Verification items for the finished model (mm, model axes). Face numbers are marked on the shaded views. A direction names the side the tool comes from. Give positions to 0.01 mm unless a question says otherwise; leave off trailing zeros. Write each loop counter-clockwise with the first axis right and the second up, starting at its lowest first coordinate (ties: lowest second). Pieces come first, ordered by that corner, then holes. Notation, with made-up numbers: M 4.5,-17.5 L 31.5,-17.5 A20 ccw 31.5,-11.5 Z; hole C 61,39.5 d3. An arc over 180 degrees is marked long. Write item = value, one per line.
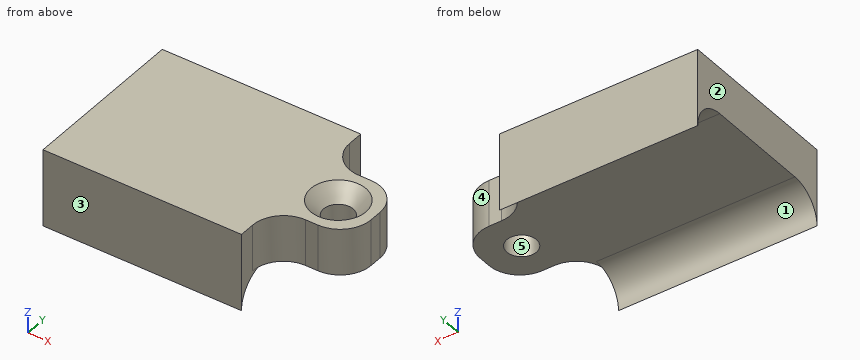
from build123d import *

# Parameters (mm, degrees)
SKETCH1_W                       = 12.8
SKETCH1_H                       = 10.8
SKETCH1_W_2                     = 4.8
SKETCH1_H_2                     = 4.8
BOSS_EXTRUDE1_DEPTH             = 1.5
F_2_CLEARANCE_HOLE1_D           = 1.905
F_2_CLEARANCE_HOLE1_CSINK_D     = 3.556
F_2_CLEARANCE_HOLE1_CSINK_ANGLE = 80
FILLET1_R                       = 2
BOSS_EXTRUDE2_REACH             = 14.524
BOSS_EXTRUDE2_DIRECTION_2_REACH = 14.524


with BuildPart() as part:
    # Sketch1 → Boss-Extrude1 (new, symmetric)
    with BuildSketch(Plane.XY):
        Rectangle(SKETCH1_W, SKETCH1_H)
        with Locations((8.8, 0)):
            Rectangle(SKETCH1_W_2, SKETCH1_H_2)
    extrude(amount=BOSS_EXTRUDE1_DEPTH, both=True)

    # #2 Clearance Hole1 (through all)
    with Locations(Plane.XY.offset(1.5)):
        with Locations((8.8, 0)):
            CounterSinkHole(F_2_CLEARANCE_HOLE1_D / 2, F_2_CLEARANCE_HOLE1_CSINK_D / 2, counter_sink_angle=F_2_CLEARANCE_HOLE1_CSINK_ANGLE)

    # Fillet1
    fillet1_edges = [part.edges().sort_by_distance(p)[0] for p in [
        (6.4, 2.4, 0),
        (11.2, 2.4, 0),
        (11.2, -2.4, 0),
        (6.4, -2.4, 0),
    ]]
    fillet(fillet1_edges, radius=FILLET1_R)

    # Boss-Extrude2: up to this face of the body (flat: up to its plane)
    boss_extrude2_end = Plane(part.part.faces().sort_by_distance((-6.4, 0, 0))[0])
    # Sketch4 → Boss-Extrude2 (add, up to the picked face)
    with BuildSketch(Plane(origin=(0, 0, 0), x_dir=(0, 0, -1), z_dir=(1, 0, 0)), mode=Mode.PRIVATE) as boss_extrude2_sk1:
        with BuildLine():
            Line((1.5, 5.4), (3.5, 5.4))
            ThreePointArc((3.5, 5.4), (2.085786438, 4.814213562), (1.5, 3.4))
            Line((1.5, 3.4), (1.5, 5.4))
        make_face()
    boss_extrude2_tool1 = split(extrude(boss_extrude2_sk1.sketch, amount=-BOSS_EXTRUDE2_REACH, mode=Mode.PRIVATE), bisect_by=boss_extrude2_end, keep=Keep.BOTH, mode=Mode.PRIVATE)
    # Sketch4 → Boss-Extrude2 (add, up to the picked face)
    with BuildSketch(Plane(origin=(0, 0, 0), x_dir=(0, 0, -1), z_dir=(1, 0, 0)), mode=Mode.PRIVATE) as boss_extrude2_sk2:
        with BuildLine():
            Line((1.5, -5.4), (1.5, -3.4))
            ThreePointArc((1.5, -3.4), (2.085786438, -4.814213562), (3.5, -5.4))
            Line((3.5, -5.4), (1.5, -5.4))
        make_face()
    boss_extrude2_tool2 = split(extrude(boss_extrude2_sk2.sketch, amount=-BOSS_EXTRUDE2_REACH, mode=Mode.PRIVATE), bisect_by=boss_extrude2_end, keep=Keep.BOTH, mode=Mode.PRIVATE)
    add(boss_extrude2_tool1.solids().sort_by(Axis((0, 4.953264, -1.946736), (-1, 0, 0)))[0])
    add(boss_extrude2_tool2.solids().sort_by(Axis((0, -4.953264, -1.946736), (-1, 0, 0)))[0])

    # Boss-Extrude2 direction 2: up to this face of the body (flat: up to its plane)
    boss_extrude2_direction_2_end = Plane(part.part.faces().sort_by_distance((6.4, 4.9, 0))[0])
    # Sketch4 → Boss-Extrude2 direction 2 (add, up to the picked face)
    with BuildSketch(Plane(origin=(0, 0, 0), x_dir=(0, 0, -1), z_dir=(1, 0, 0)), mode=Mode.PRIVATE) as boss_extrude2_direction_2_sk1:
        with BuildLine():
            Line((1.5, 5.4), (3.5, 5.4))
            ThreePointArc((3.5, 5.4), (2.085786438, 4.814213562), (1.5, 3.4))
            Line((1.5, 3.4), (1.5, 5.4))
        make_face()
    boss_extrude2_direction_2_tool1 = split(extrude(boss_extrude2_direction_2_sk1.sketch, amount=BOSS_EXTRUDE2_DIRECTION_2_REACH, mode=Mode.PRIVATE), bisect_by=boss_extrude2_direction_2_end, keep=Keep.BOTH, mode=Mode.PRIVATE)
    # Sketch4 → Boss-Extrude2 direction 2 (add, up to the picked face)
    with BuildSketch(Plane(origin=(0, 0, 0), x_dir=(0, 0, -1), z_dir=(1, 0, 0)), mode=Mode.PRIVATE) as boss_extrude2_direction_2_sk2:
        with BuildLine():
            Line((1.5, -5.4), (1.5, -3.4))
            ThreePointArc((1.5, -3.4), (2.085786438, -4.814213562), (3.5, -5.4))
            Line((3.5, -5.4), (1.5, -5.4))
        make_face()
    boss_extrude2_direction_2_tool2 = split(extrude(boss_extrude2_direction_2_sk2.sketch, amount=BOSS_EXTRUDE2_DIRECTION_2_REACH, mode=Mode.PRIVATE), bisect_by=boss_extrude2_direction_2_end, keep=Keep.BOTH, mode=Mode.PRIVATE)
    add(boss_extrude2_direction_2_tool1.solids().sort_by(Axis((0, 4.953264, -1.946736), (1, 0, 0)))[0])
    add(boss_extrude2_direction_2_tool2.solids().sort_by(Axis((0, -4.953264, -1.946736), (1, 0, 0)))[0])


solid = part.part
1) Draft check along X on the marked faces 3, 4 and 5. Enter one of: +X half, -X half, draft (parallel to the pull), parting line (faces both ways), or undercut.
From the geometry:
face_3 = draft
face_4 = +X half
face_5 = undercut
2) Tool access check on the marked faces 1 and 2. Record the directions out of +Z, -Z, +X, -X, +Y, -Y that give a thin tool (end or side, any length) a straight path to the whole face; none if there is none.
From the geometry:
face_1 = -Z, +X, -X
face_2 = +Z, -Z, -X, +Y, -Y
3) Cross-section at D-D on x = -1.75. Record the boundary of the cut face in (y, z), plus the area to 3 significant figures.
From the geometry:
outline = M -5.4,-3.5 A2 cw -3.4,-1.5 L 3.4,-1.5 A2 cw 5.4,-3.5 L 5.4,1.5 L -5.4,1.5 Z
area = 34.1 mm^2
4) Cross-section at A-A on x = 8.8. Record the boundary of the cut face in (y, z).
From the geometry:
outline = M -2.4,-1.5 L -0.95,-1.5 L -0.95,0.52 L -1.78,1.5 L -2.4,1.5 Z; M 0.95,-1.5 L 2.4,-1.5 L 2.4,1.5 L 1.78,1.5 L 0.95,0.52 Z
5) Depth check by flat-ended pin: P1, Ø4.5, axis at x = 4, y = 0.5, coming from the -Z side; P2, Ø1.6, axis at y = -5, z = 0, coming from the +X side; P3, Ø2, axis at x = 6.5, z = -1, coming from the +Y side; P4, Ø1.5, axis at y = 2, z = -0.5, coming from the +X side. Enter the tip coordinate at first touch or a pass-through.
From the geometry:
P1 = -1.5
P2 = 6.41
P3 = 5.4
P4 = 11.01
6) Material ranges on probe 1 along X at (y, z) = (0, -0.55); probe 2 along Y at (x, z) = (8.8, -0.6); probe 3 along Y at (x, z) = (2.25, -2.2), recorded low to high. Write a range as from..to.
From the geometry:
probe_1 = -6.4..7.85, 9.75..11.2
probe_2 = -2.4..-0.95, 0.95..2.4
probe_3 = -5.4..-4.92, 4.92..5.4
7) Cross-section at B-B on z = -0.6. Record the boundary of the cut face in (x, y) (1 decimal).
From the geometry:
outline = M -6.4,-5.4 L 6.4,-5.4 L 6.4,-4.4 A2 cw 8.4,-2.4 L 9.2,-2.4 A2 ccw 11.2,-0.4 L 11.2,0.4 A2 ccw 9.2,2.4 L 8.4,2.4 A2 cw 6.4,4.4 L 6.4,5.4 L -6.4,5.4 Z; hole C 8.8,0 d1.9
8) Cross-section at C-C on z = -2.9. Record the boundary of the cut face in (x, y).
From the geometry:
outline = M -6.4,-5.4 L 6.4,-5.4 L 6.4,-5.31 L -6.4,-5.31 Z; M -6.4,5.31 L 6.4,5.31 L 6.4,5.4 L -6.4,5.4 Z
